Can you work these out from the model? Positions are in its coordinate system, mm. A direction names the side the tool comes from. Round coordinates to 2 decimals unless told otherwise and drop trailing zeros. Write item = value, one per line. Start each with the question number.
1) For faces 1 (the face through (4.27, 5.33, -101.4)), 2 (the face through (2.4, 0.1, 0)), 3 (the face through (-10, 6, -101)), 4 (the face through (3.655, 0, -101)), 5 (the face through (0, -3.655, -101)), which set-ups out of +Z, -Z, +X, -X, +Y, -Y let a thin tool reach every point of the face, with its end or its side?
2) I'm going to push flat-ended pins straight in: pin 1 (4 mm diameter, centred on y = 0, z = -122, fed in from -X) (3 decimals); pin 2 (0.5 mm diameter, centred on y = -9, z = -124.5, fed in from -X). Where does each tip first touch, or does it pass through?
3) If I drill on line 1 (X direction, y = 7.5, z = -180.5) (3 decimals); line 2 (Y direction, x = -3.75, z = -22); line 3 (X direction, y = 0.75, z = -120.5) (3 decimals), over which ranges is the centre line in solid material (lowest first)?
4) Thinking about a two-plate mould opening in Y: for faces 6 (the face through (0, 3.655, -101)), 7 (the face through (6, -10, -101)), 8 (the face through (5.33, -4.27, -101.4)), 9 (the face through (2.4, 0.1, -200)), which applies, +Y half, -Y half, draft (parallel to the pull), parting line (faces both ways), or undercut?
from build123d import *

# Parameters (mm, degrees)
BOSS_EXTRUDE1_DEPTH = 200


with BuildPart() as part:
    # Sketch1 → Boss-Extrude1 (new body)
    with BuildSketch(Plane(origin=(0, 0, -200), x_dir=(-1, 0, 0), z_dir=(0, 0, -1))):
        with BuildLine():
            Line((10, -8.5), (10, -3.138))
            ThreePointArc((10, -3.138), (9.851210245, -2.778789755), (9.492, -2.63))
            Line((9.492, -2.63), (9.008, -2.63))
            ThreePointArc((9.008, -2.63), (8.648789755, -2.778789755), (8.5, -3.138))
            Line((8.5, -3.138), (8.5, -5.487))
            ThreePointArc((8.5, -5.487), (8.351210245, -5.846210245), (7.992, -5.995))
            Line((7.992, -5.995), (7.26592049, -5.995))
            ThreePointArc((7.26592049, -5.995), (7.071517306, -5.956330803), (6.906710245, -5.846210245))
            Line((6.906710245, -5.846210245), (3.803789755, -2.743289755))
            ThreePointArc((3.803789755, -2.743289755), (3.693669197, -2.578482694), (3.655, -2.38407951))
            Line((3.655, -2.38407951), (3.655, 2.383759167))
            ThreePointArc((3.655, 2.383759167), (3.693669197, 2.57816235), (3.803789755, 2.742969412))
            Line((3.803789755, 2.742969412), (6.907030588, 5.846210245))
            ThreePointArc((6.907030588, 5.846210245), (7.07183765, 5.956330803), (7.266240833, 5.995))
            Line((7.266240833, 5.995), (7.992, 5.995))
            ThreePointArc((7.992, 5.995), (8.351210245, 5.846210245), (8.5, 5.487))
            Line((8.5, 5.487), (8.5, 3.138))
            ThreePointArc((8.5, 3.138), (8.648789755, 2.778789755), (9.008, 2.63))
            Line((9.008, 2.63), (9.492, 2.63))
            ThreePointArc((9.492, 2.63), (9.851210245, 2.778789755), (10, 3.138))
            Line((10, 3.138), (10, 8.5))
            ThreePointArc((10, 8.5), (9.560660172, 9.560660172), (8.5, 10))
            Line((8.5, 10), (3.138, 10))
            ThreePointArc((3.138, 10), (2.778789755, 9.851210245), (2.63, 9.492))
            Line((2.63, 9.492), (2.63, 9.008))
            ThreePointArc((2.63, 9.008), (2.778789755, 8.648789755), (3.138, 8.5))
            Line((3.138, 8.5), (5.487, 8.5))
            ThreePointArc((5.487, 8.5), (5.846210245, 8.351210245), (5.995, 7.992))
            Line((5.995, 7.992), (5.995, 7.26592049))
            ThreePointArc((5.995, 7.26592049), (5.956330803, 7.071517306), (5.846210245, 6.906710245))
            Line((5.846210245, 6.906710245), (2.743289755, 3.803789755))
            ThreePointArc((2.743289755, 3.803789755), (2.578482694, 3.693669197), (2.38407951, 3.655))
            Line((2.38407951, 3.655), (-2.383759167, 3.655))
            ThreePointArc((-2.383759167, 3.655), (-2.57816235, 3.693669197), (-2.742969412, 3.803789755))
            Line((-2.742969412, 3.803789755), (-5.846210245, 6.907030588))
            ThreePointArc((-5.846210245, 6.907030588), (-5.956330803, 7.07183765), (-5.995, 7.266240833))
            Line((-5.995, 7.266240833), (-5.995, 7.992))
            ThreePointArc((-5.995, 7.992), (-5.846210245, 8.351210245), (-5.487, 8.5))
            Line((-5.487, 8.5), (-3.138, 8.5))
            ThreePointArc((-3.138, 8.5), (-2.778789755, 8.648789755), (-2.63, 9.008))
            Line((-2.63, 9.008), (-2.63, 9.492))
            ThreePointArc((-2.63, 9.492), (-2.778789755, 9.851210245), (-3.138, 10))
            Line((-3.138, 10), (-8.5, 10))
            ThreePointArc((-8.5, 10), (-9.560660172, 9.560660172), (-10, 8.5))
            Line((-10, 8.5), (-10, 3.138))
            ThreePointArc((-10, 3.138), (-9.851210245, 2.778789755), (-9.492, 2.63))
            Line((-9.492, 2.63), (-9.008, 2.63))
            ThreePointArc((-9.008, 2.63), (-8.648789755, 2.778789755), (-8.5, 3.138))
            Line((-8.5, 3.138), (-8.5, 5.487))
            ThreePointArc((-8.5, 5.487), (-8.351210245, 5.846210245), (-7.992, 5.995))
            Line((-7.992, 5.995), (-7.26592049, 5.995))
            ThreePointArc((-7.26592049, 5.995), (-7.071517306, 5.956330803), (-6.906710245, 5.846210245))
            Line((-6.906710245, 5.846210245), (-3.803789755, 2.743289755))
            ThreePointArc((-3.803789755, 2.743289755), (-3.693669197, 2.578482694), (-3.655, 2.38407951))
            Line((-3.655, 2.38407951), (-3.655, -2.383759167))
            ThreePointArc((-3.655, -2.383759167), (-3.693669197, -2.57816235), (-3.803789755, -2.742969412))
            Line((-3.803789755, -2.742969412), (-6.907030588, -5.846210245))
            ThreePointArc((-6.907030588, -5.846210245), (-7.07183765, -5.956330803), (-7.266240833, -5.995))
            Line((-7.266240833, -5.995), (-7.992, -5.995))
            ThreePointArc((-7.992, -5.995), (-8.351210245, -5.846210245), (-8.5, -5.487))
            Line((-8.5, -5.487), (-8.5, -3.138))
            ThreePointArc((-8.5, -3.138), (-8.648789755, -2.778789755), (-9.008, -2.63))
            Line((-9.008, -2.63), (-9.492, -2.63))
            ThreePointArc((-9.492, -2.63), (-9.851210245, -2.778789755), (-10, -3.138))
            Line((-10, -3.138), (-10, -8.5))
            ThreePointArc((-10, -8.5), (-9.560660172, -9.560660172), (-8.5, -10))
            Line((-8.5, -10), (-3.138, -10))
            ThreePointArc((-3.138, -10), (-2.778789755, -9.851210245), (-2.63, -9.492))
            Line((-2.63, -9.492), (-2.63, -9.008))
            ThreePointArc((-2.63, -9.008), (-2.778789755, -8.648789755), (-3.138, -8.5))
            Line((-3.138, -8.5), (-5.487, -8.5))
            ThreePointArc((-5.487, -8.5), (-5.846210245, -8.351210245), (-5.995, -7.992))
            Line((-5.995, -7.992), (-5.995, -7.26592049))
            ThreePointArc((-5.995, -7.26592049), (-5.956330803, -7.071517306), (-5.846210245, -6.906710245))
            Line((-5.846210245, -6.906710245), (-2.743289755, -3.803789755))
            ThreePointArc((-2.743289755, -3.803789755), (-2.578482694, -3.693669197), (-2.38407951, -3.655))
            Line((-2.38407951, -3.655), (2.383759167, -3.655))
            ThreePointArc((2.383759167, -3.655), (2.57816235, -3.693669197), (2.742969412, -3.803789755))
            Line((2.742969412, -3.803789755), (5.846210245, -6.907030588))
            ThreePointArc((5.846210245, -6.907030588), (5.956330803, -7.07183765), (5.995, -7.266240833))
            Line((5.995, -7.266240833), (5.995, -7.992))
            ThreePointArc((5.995, -7.992), (5.846210245, -8.351210245), (5.487, -8.5))
            Line((5.487, -8.5), (3.138, -8.5))
            ThreePointArc((3.138, -8.5), (2.778789755, -8.648789755), (2.63, -9.008))
            Line((2.63, -9.008), (2.63, -9.492))
            ThreePointArc((2.63, -9.492), (2.778789755, -9.851210245), (3.138, -10))
            Line((3.138, -10), (8.5, -10))
            ThreePointArc((8.5, -10), (9.560660172, -9.560660172), (10, -8.5))
        make_face()
        with BuildLine():
            Line((2.304493037, -2.124493037), (2.124493037, -2.304493037))
            ThreePointArc((2.124493037, -2.304493037), (1.35638567, -2.506016078), (0.803729988, -1.935777391))
            ThreePointArc((0.803729988, -1.935777391), (0, -2.096), (-0.803729988, -1.935777391))
            ThreePointArc((-0.803729988, -1.935777391), (-1.35638567, -2.506016078), (-2.124493037, -2.304493037))
            Line((-2.124493037, -2.304493037), (-2.304493037, -2.124493037))
            ThreePointArc((-2.304493037, -2.124493037), (-2.506016078, -1.35638567), (-1.935777391, -0.803729988))
            ThreePointArc((-1.935777391, -0.803729988), (-2.096, 0), (-1.935777391, 0.803729988))
            ThreePointArc((-1.935777391, 0.803729988), (-2.506016078, 1.35638567), (-2.304493037, 2.124493037))
            Line((-2.304493037, 2.124493037), (-2.124493037, 2.304493037))
            ThreePointArc((-2.124493037, 2.304493037), (-1.35638567, 2.506016078), (-0.803729988, 1.935777391))
            ThreePointArc((-0.803729988, 1.935777391), (0, 2.096), (0.803729988, 1.935777391))
            ThreePointArc((0.803729988, 1.935777391), (1.35638567, 2.506016078), (2.124493037, 2.304493037))
            Line((2.124493037, 2.304493037), (2.304493037, 2.124493037))
            ThreePointArc((2.304493037, 2.124493037), (2.506016078, 1.35638567), (1.935777391, 0.803729988))
            ThreePointArc((1.935777391, 0.803729988), (2.096, 0), (1.935777391, -0.803729988))
            ThreePointArc((1.935777391, -0.803729988), (2.506016078, -1.35638567), (2.304493037, -2.124493037))
        make_face(mode=Mode.SUBTRACT)
    extrude(amount=-BOSS_EXTRUDE1_DEPTH)


solid = part.part
Reported:
q1.face_1 = +Z, -Z
q1.face_2 = +Z, +X, -X, +Y, -Y
q1.face_3 = +Z, -Z, -X, +Y, -Y
q1.face_4 = +Z, -Z, +X
q1.face_5 = +Z, -Z, -Y
q2.pin_1 = -3.655
q2.pin_2 = -9.98
q3.line_1 = -10 to -5.995, 5.995 to 10
q3.line_2 = -10 to -8.5, -4.81 to -2.68, 2.68 to 4.81, 8.5 to 10
q3.line_3 = -3.655 to -1.957, 1.957 to 3.655
q4.face_6 = +Y half
q4.face_7 = -Y half
q4.face_8 = undercut
q4.face_9 = draft
